Can you work these out from the model? Positions are in its coordinate system, mm. Face numbers are marked on the shaded views. Give positions to 0.01 mm unless a question says otherwise; leave off trailing zeros. Order: outer loops, then holes, each group sorted by start corner. A loop starts at its lowest first (then second) coordinate and runs counter-clockwise, first axis right, second up.
```python
from build123d import *

# Parameters (mm, degrees)
SKETCH1_R           = 11.7
SKETCH1_R_2         = 11.075
BOSS_EXTRUDE1_DEPTH = 1.4
SKETCH1_3_R         = 0.2
SKETCH1_3_R_2       = 2.5
SKETCH1_3_R_3       = 0.7
BOSS_EXTRUDE2_DEPTH = 0.45


with BuildPart() as part:
    # Sketch1 → Boss-Extrude1 (new body)
    with BuildSketch(Plane.XY):
        Circle(SKETCH1_R)
        Circle(SKETCH1_R_2, mode=Mode.SUBTRACT)
    extrude(amount=BOSS_EXTRUDE1_DEPTH)

    # Sketch1_3 → Boss-Extrude2 (add)
    # profile 1 of 5: a face of its own
    with BuildSketch(Plane.XY):
        with BuildLine():
            Line((0.6, 2.42693222), (0.6, 11.058735235))
            ThreePointArc((0.6, 11.058735235), (0, 11.075), (-0.6, 11.058735235))
            Line((-0.6, 11.058735235), (-0.6, 2.42693222))
            ThreePointArc((-0.6, 2.42693222), (0, 2.5), (0.6, 2.42693222))
        make_face()
        with Locations((0, 9.5)):
            Circle(SKETCH1_3_R, mode=Mode.SUBTRACT)
    # profile 2 of 5: a face of its own
    with BuildSketch(Plane.XY):
        with BuildLine():
            Line((-2.42693222, 0.6), (-11.058735235, 0.6))
            ThreePointArc((-11.058735235, 0.6), (-11.075, 0), (-11.058735235, -0.6))
            Line((-11.058735235, -0.6), (-2.42693222, -0.6))
            ThreePointArc((-2.42693222, -0.6), (-2.5, 0), (-2.42693222, 0.6))
        make_face()
        with Locations((-9.5, 0)):
            Circle(SKETCH1_3_R, mode=Mode.SUBTRACT)
    # profile 3 of 5: a face of its own
    with BuildSketch(Plane.XY):
        with BuildLine():
            ThreePointArc((11.075, 0), (11.070933062, 0.300110206), (11.058735235, 0.6))
            Line((11.058735235, 0.6), (2.42693222, 0.6))
            ThreePointArc((2.42693222, 0.6), (2.481665827, 0.302216355), (2.5, 0))
            ThreePointArc((2.5, 0), (2.481665827, -0.302216355), (2.42693222, -0.6))
            Line((2.42693222, -0.6), (11.058735235, -0.6))
            ThreePointArc((11.058735235, -0.6), (11.070933062, -0.300110206), (11.075, 0))
        make_face()
        with Locations((9.5, 0)):
            Circle(SKETCH1_3_R, mode=Mode.SUBTRACT)
    # profile 4 of 5: a face of its own
    with BuildSketch(Plane.XY):
        Circle(SKETCH1_3_R_2)
        Circle(SKETCH1_3_R_3, mode=Mode.SUBTRACT)
    # profile 5 of 5: a face of its own
    with BuildSketch(Plane.XY):
        with BuildLine():
            ThreePointArc((-0.6, -11.058735235), (0, -11.075), (0.6, -11.058735235))
            Line((0.6, -11.058735235), (0.6, -2.42693222))
            ThreePointArc((0.6, -2.42693222), (0, -2.5), (-0.6, -2.42693222))
            Line((-0.6, -2.42693222), (-0.6, -11.058735235))
        make_face()
        with Locations((0, -9.5)):
            Circle(SKETCH1_3_R, mode=Mode.SUBTRACT)
    extrude(amount=BOSS_EXTRUDE2_DEPTH)


solid = part.part
```
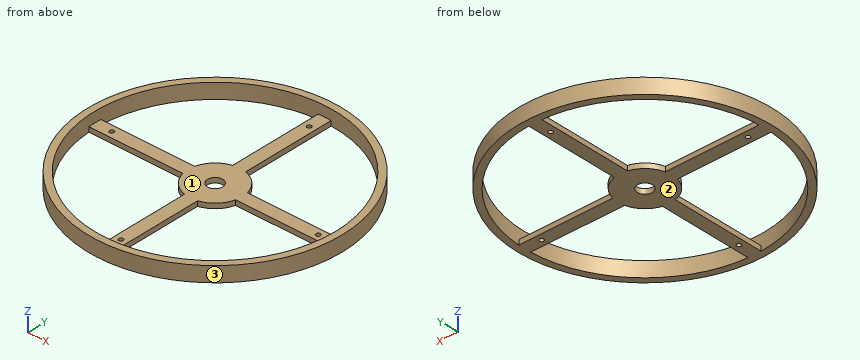
1) Suppose I cut it at A-A (y = -10). Please give me the cut outline in (x, z).
2) Suppose I cut it at C-C (z = 0.7). Please give me the cut outline in (x, y) (3 decimals).
3) Suppose I cut it at B-B (x = 1). Please give me the cut outline in (y, z), and give its area (3 significant figures).
4) I'm going to push flat-ended pins straight in: pin 1 Ø0.8 at (x, y) = (0, 0) entering from -Z; pin 2 Ø0.5 at (x, z) = (-8, 0.5) entering from -Y; pin 3 Ø6.5 at (x, y) = (-2.5, 1) entering from +Z. Where does each tip first touch, or does it pass through?
5) We'd pull the mould along X, two halves only. Please class the marked faces 1, 2 and 3: +X half, -X half, draft (parallel to the pull), parting line (faces both ways), or undercut.
6) If I drill on line 1 (Y direction, x = 0, z = 0.35); line 2 (Y direction, x = 0, z = 0.7) (3 decimals); line 3 (Y direction, x = 2, z = 0.15), over which ranges is the centre line in solid material (lowest first)?
Results:
1. outline: (-6.07, 0) - (-4.76, 0) - (-4.76, 1.4) - (-6.07, 1.4) - close; (-0.6, 0) - (0.6, 0) - (0.6, 0.45) - (-0.6, 0.45) - close; (4.76, 0) - (6.07, 0) - (6.07, 1.4) - (4.76, 1.4) - close
2. outline: circle Ø23.4 at (0, 0); hole circle Ø22.15 at (0, 0)
3. outline: (-11.66, 0) - (-11.03, 0) - (-11.03, 1.4) - (-11.66, 1.4) - close; (-2.29, 0) - (2.29, 0) - (2.29, 0.45) - (-2.29, 0.45) - close; (11.03, 0) - (11.66, 0) - (11.66, 1.4) - (11.03, 1.4) - close
3. area: 3.82 mm2
4. pin 1: passes through
4. pin 2: stops at y = -8.77
4. pin 3: stops at z = 0.45
5. face 1: undercut
5. face 2: draft
5. face 3: parting line
6. line 1: y = -11.7 to -9.7, -9.3 to -0.7, 0.7 to 9.3, 9.7 to 11.7
6. line 2: y = -11.7 to -11.075, 11.075 to 11.7
6. line 3: y = -11.53 to -10.89, -1.5 to 1.5, 10.89 to 11.53
